Check sheet for the modelled part. Datum: model origin and axes. Units: mm. A direction names the side the tool comes from. Round coordinates to 2 decimals unless told otherwise and drop trailing zeros. Order: outer loops, then holes, each group sorted by start corner. A loop starts at its lowest first (then second) coordinate and runs counter-clockwise, first axis right, second up. Notation, with made-up numbers: M -28,83.5 L -6,83.5 A36 cw -6,122.5 Z; hole C 64,87.5 d2. An arc over 180 degrees is marked long. One line per item, written item: value. Start each with the question number.
(1) Depth check by flat-ended pin: pin 1 Ø2 at (x, z) = (-23, 16.5) entering from -Y; pin 2 Ø8 at (x, z) = (-22.5, 17.5) entering from +Y. Enter the tip coordinate at first touch or a pass-through.
(2) Thickness scan on L1, parallel to X at y = 16.25, z = 9.75; L2, parallel to Y at x = -21.75, z = 18.5; L3, parallel to Y at x = -16.25, z = 19.5. Record the ranges inside material, lowest first.
(3) Access from +Z, -Z, +X, -X, +Y, -Y to the whole of each face (thin tool, end or side, straight path). Record for faces 1 (the face through (-22.4, 15.07, 12.32)), 2 (the face through (-8, 25, 12)).
(4) Cross-section at C-C, the plane x = -16. Enter the section's corners in (y, z).
(5) Cross-section at A-A, the plane z = 9.75. Enter the section's corners in (x, y), and give its area (4 significant figures).
(6) Cross-section at B-B, the plane y = 14.5. Enter the section's corners in (x, z).
from build123d import *

# Parameters (mm, degrees)
BOSS_EXTRUDE1_DEPTH = 25
BOSS_EXTRUDE4_DEPTH = 15


with BuildPart() as part:
    # Sketch1 → Boss-Extrude1 (new body)
    with BuildSketch(Plane.XY):
        Polygon((-15, 25), (0, 25), (0, 0), (-30, 0), (-30, 10), (-15, 10), align=None)
    extrude(amount=BOSS_EXTRUDE1_DEPTH)

    # Sketch5 → Boss-Extrude4 (add)
    with BuildSketch(Plane.ZY.offset(15)):
        Polygon((0, 10), (0, 20), (25, 10), align=None)
    extrude(amount=BOSS_EXTRUDE4_DEPTH)


solid = part.part
Values found:
1. pin 1: y = 0
1. pin 2: y = 14.6
2. L1: -15 to 0
2. L2: 0 to 12.6
2. L3: 0 to 12.2
3. face 1: +Z, -X, +Y
3. face 2: +Z, -Z, +X, -X, +Y
4. outline: M 0,0 L 20,0 L 10,25 L 0,25 Z
5. outline: M -30,0 L 0,0 L 0,25 L -15,25 L -15,16.1 L -30,16.1 Z
5. area: 616.5 mm^2
6. outline: M -30,0 L 0,0 L 0,25 L -15,25 L -15,13.75 L -30,13.75 Z
